```python
from build123d import *

# Parameters (mm, degrees)
EXTRUDE_1_DEPTH     = 4
SKETCH_2_W          = 5.98
SKETCH_2_H          = 10
EXTRUDE_2_DEPTH     = 4
SKETCH_4_R          = 1
SKETCH_4_W          = 55
SKETCH_4_H          = 8
CUT_EXTRUDE_1_DEPTH = 4
SKETCH_5_R          = 1.6
CUT_EXTRUDE_2_DEPTH = 4
SKETCH_6_W          = 31.5
SKETCH_6_H          = 52
EXTRUDE_3_DEPTH     = 4
SKETCH_7_R          = 1.6
CUT_EXTRUDE_3_DEPTH = 4
SKETCH_8_W          = 13.057041555
SKETCH_8_H          = 52
SKETCH_8_W_2        = 44.99
SKETCH_8_H_2        = 3
EXTRUDE_4_DEPTH     = 4
SKETCH_10_R         = 2.05
CUT_EXTRUDE_4_DEPTH = 10
FILLET_1_R          = 1
FILLET_2_R          = 3
SKETCH_11_W         = 28.99
SKETCH_11_H         = 30
CUT_EXTRUDE_5_DEPTH = 10
EXTRUDE_1_2_DEPTH   = 4
FILLET_3_R          = 2
SKETCH_13_R         = 1.6
EXTRUDE_5_DEPTH     = 4
SKETCH_15_R         = 1.6
CUT_EXTRUDE_6_DEPTH = 4


with BuildPart() as part:
    # 草图1 → Extrude 1 (new body)
    with BuildSketch(Plane(origin=(0, 0, 0), x_dir=(1, 0, 0), z_dir=(0, 1, 0))):
        Polygon((-14.01, 30), (-27.5, 30), (-27.5, -30), (27.5, -30), (27.5, 30), (14.01, 30), (14.01, 22), (14.01, -22), (-14.01, -22), (-14.01, 22), align=None)
    extrude(amount=EXTRUDE_1_DEPTH)

    # 草图2 → 凸台-拉伸2 (add)
    with BuildSketch(Plane(origin=(0, 4, 0), x_dir=(1, 0, 0), z_dir=(0, 1, 0))):
        with Locations((-6, -17)):
            Rectangle(SKETCH_2_W, SKETCH_2_H)
        with Locations((6, -17)):
            Rectangle(SKETCH_2_W, SKETCH_2_H)
    extrude(amount=-EXTRUDE_2_DEPTH)

    # 草图4 → 切除-拉伸1 (cut)
    with BuildSketch(Plane.XZ):
        with Locations((8.99, 21)):
            Circle(SKETCH_4_R)
        with Locations((14.01, 21)):
            Circle(SKETCH_4_R)
        with Locations((-2.01, 22)):
            Circle(SKETCH_4_R)
        with Locations((2.01, 22)):
            Circle(SKETCH_4_R)
        with Locations((-14.01, 21)):
            Circle(SKETCH_4_R)
        with Locations((-8.99, 21)):
            Circle(SKETCH_4_R)
        with Locations((0, -26)):
            Rectangle(SKETCH_4_W, SKETCH_4_H)
    extrude(amount=-CUT_EXTRUDE_1_DEPTH, mode=Mode.SUBTRACT)

    # 草图5 → 切除-拉伸2 (cut)
    with BuildSketch(Plane.XZ):
        with Locations(Location((17.01, 10, 0), (0, 0, 270))):
            Circle(SKETCH_5_R)
        with Locations(Location((17.01, -10, 0), (0, 0, 270))):
            Circle(SKETCH_5_R)
        with Locations(Location((-17.01, -10, 0), (0, 0, 270))):
            Circle(SKETCH_5_R)
        with Locations(Location((-17.01, 10, 0), (0, 0, 270))):
            Circle(SKETCH_5_R)
    extrude(amount=-CUT_EXTRUDE_2_DEPTH, mode=Mode.SUBTRACT)

    # 草图6 → 凸台-拉伸3 (add)
    with BuildSketch(Plane.XZ):
        with Locations((43.25, 4)):
            Rectangle(SKETCH_6_W, SKETCH_6_H)
    extrude(amount=-EXTRUDE_3_DEPTH)

    # 草图7 → 切除-拉伸3 (cut)
    with BuildSketch(Plane.XZ):
        with Locations(Location((56, 20, 0), (0, 0, 270))):
            Circle(SKETCH_7_R)
        with Locations(Location((56, 0, 0), (0, 0, 270))):
            Circle(SKETCH_7_R)
    extrude(amount=-CUT_EXTRUDE_3_DEPTH, mode=Mode.SUBTRACT)

    # 草图8 → 凸台-拉伸4 (add)
    with BuildSketch(Plane.XZ):
        with Locations((-34.028520778, 4)):
            Rectangle(SKETCH_8_W, SKETCH_8_H)
        Polygon((-14.01, -25), (-14.01, -22), (-27.5, -22), (-40.557041555, -22), (-40.557041555, -25), align=None)
        with Locations((36.505, -23.5)):
            Rectangle(SKETCH_8_W_2, SKETCH_8_H_2)
    extrude(amount=-EXTRUDE_4_DEPTH)

    # 草图10 → 切除-拉伸4 (cut)
    with BuildSketch(Plane.XZ):
        with Locations(Location((-35.507041555, -20.5, 0), (0, 0, 270))):
            Circle(SKETCH_10_R)
        with Locations(Location((-35.507041555, 20.5, 0), (0, 0, 270))):
            Circle(SKETCH_10_R)
        with Locations(Location((35.507041555, 20.5, 0), (0, 0, 270))):
            Circle(SKETCH_10_R)
        with Locations(Location((35.507041555, -20.5, 0), (0, 0, 270))):
            Circle(SKETCH_10_R)
    extrude(amount=-CUT_EXTRUDE_4_DEPTH, mode=Mode.SUBTRACT)

    # 圆角1
    fillet_1_edges = [part.edges().sort_by_distance(p)[0] for p in [
        (-8.99, 2, 12),
        (-3.01, 2, 12),
        (3.01, 2, 12),
        (8.99, 2, 12),
    ]]
    fillet(fillet_1_edges, radius=FILLET_1_R)

    # 圆角2
    fillet_2_edges = [part.edges().sort_by_distance(p)[0] for p in [
        (59, 2, 30),
        (-40.557041555, 2, -25),
        (-14.01, 2, -25),
        (-40.557041555, 2, 30),
        (14.01, 2, -25),
        (59, 2, -25),
    ]]
    fillet(fillet_2_edges, radius=FILLET_2_R)

    # 草图11 → 切除-拉伸5 (cut)
    with BuildSketch(Plane(origin=(0, 4, 0), x_dir=(1, 0, 0), z_dir=(0, 1, 0))):
        with Locations((36.505, 0)):
            Rectangle(SKETCH_11_W, SKETCH_11_H)
        with BuildLine():
            Line((-23, 11), (-23, -11))
            ThreePointArc((-23, -11), (-28, -16), (-33, -11))
            Line((-33, -11), (-33, 11))
            ThreePointArc((-33, 11), (-28, 16), (-23, 11))
        make_face()
    extrude(amount=-CUT_EXTRUDE_5_DEPTH, mode=Mode.SUBTRACT)

    # 草图12 → Extrude 1 2 (add)
    with BuildSketch(Plane(origin=(0, 4, 0), x_dir=(1, 0, 0), z_dir=(0, 1, 0))):
        Polygon((20.571783704, 13.610203653), (49.561783704, -16.389796347), (52.438216296, -13.610203653), (23.448216296, 16.389796347), align=None)
        Polygon((23.448216296, -16.389796347), (52.438216296, 13.610203653), (49.561783704, 16.389796347), (20.571783704, -13.610203653), align=None)
    extrude(amount=-EXTRUDE_1_2_DEPTH)

    # 圆角3
    fillet_3_edges = [part.edges().sort_by_distance(p)[0] for p in [
        (24.791222833, 2, 15),
        (48.218777167, 2, 15),
        (51, 2, -12.121880477),
        (51, 2, 12.121880477),
        (48.218777167, 2, -15),
        (24.791222833, 2, -15),
        (22.01, 2, 12.121880477),
        (22.01, 2, -12.121880477),
        (33.723777167, 2, 0),
        (36.505, 2, -2.878119523),
        (39.286222833, 2, 0),
        (36.505, 2, 2.878119523),
    ]]
    fillet(fillet_3_edges, radius=FILLET_3_R)

    # 草图13 → 凸台-拉伸5 (add)
    with BuildSketch(Plane.XZ):
        with Locations((17.01, -10)):
            Circle(SKETCH_13_R)
        with Locations((17.01, 10)):
            Circle(SKETCH_13_R)
        with Locations((-17.01, -10)):
            Circle(SKETCH_13_R)
        with Locations((-17.01, 10)):
            Circle(SKETCH_13_R)
    extrude(amount=-EXTRUDE_5_DEPTH)

    # 草图15 → 切除-拉伸6 (cut)
    with BuildSketch(Plane.XZ):
        with Locations(Location((-17.320508076, -10, 0), (0, 0, 270))):
            Circle(SKETCH_15_R)
        with Locations(Location((-17.320508076, 10, 0), (0, 0, 270))):
            Circle(SKETCH_15_R)
        with Locations(Location((17.320508076, 10, 0), (0, 0, 270))):
            Circle(SKETCH_15_R)
        with Locations(Location((17.320508076, -10, 0), (0, 0, 270))):
            Circle(SKETCH_15_R)
    extrude(amount=-CUT_EXTRUDE_6_DEPTH, mode=Mode.SUBTRACT)


solid = part.part
```
Check sheet for the modelled part. Datum: model origin and axes. Units: mm. A direction names the side the tool comes from. Round coordinates to 2 decimals unless told otherwise and drop trailing zeros. Order: outer loops, then holes, each group sorted by start corner. A loop starts at its lowest first (then second) coordinate and runs counter-clockwise, first axis right, second up. Notation, with made-up numbers: M -6,7.5 L 40,7.5 A21 cw 40,35.5 Z; hole C -16,70.5 d7. An arc over 180 degrees is marked long. Answer in a Markdown table with one row per item.
(1) Section check A-A on z = 0. Record the boundary of the cut face in (x, y), plus the area to 3 significant figures.
Findings:
| item | result |
|---|---|
| outline | M -40.56,0 L -33,0 L -33,4 L -40.56,4 Z; M -23,0 L -14.01,0 L -14.01,4 L -23,4 Z; M 14.01,0 L 22.01,0 L 22.01,4 L 14.01,4 Z; M 32.94,0 L 40.07,0 L 40.07,4 L 32.94,4 Z; M 51,0 L 54.4,0 L 54.4,4 L 51,4 Z; M 57.6,0 L 59,0 L 59,4 L 57.6,4 Z |
| area | 146 mm^2 |
(2) Material ranges on line 1 along X through (y, z) = (1.6, 16.5); line 2 along X through (y, z) = (2.4, 13.5); line 3 along X through (y, z) = (1.55, 10), recorded low to high. Write a range as from..to.
Findings:
| item | result |
|---|---|
| line 1 | x = -40.56..-14.01, -8.99..-3.01, 3.01..8.99, 14.01..59 |
| line 2 | x = -40.56..-32.33, -23.67..-14.01, -8.99..-3.01, 3.01..8.99, 14.01..27.57, 45.44..59 |
| line 3 | x = -40.56..-33, -23..-18.92, -15.72..-14.01, 14.01..15.72, 18.92..29.62, 43.39..59 |
(3) Draft check along Z on faces 1 (the cylindrical face through (37.54, 1.97, 20.77)), 2 (the flat face through (14.01, 2, -1)), 3 (the flat face through (12, 2, 22)). Enter one of: +Z half, -Z half, draft (parallel to the pull), parting line (faces both ways), or undercut.
Findings:
| item | result |
|---|---|
| face 1 | undercut |
| face 2 | draft |
| face 3 | -Z half |
(4) Gauge pin test, flat ends, axial feed: pin 1 (4.5 mm diameter, centred on x = 35.51, z = -20.5, fed in from +Y); pin 2 (2.5 mm diameter, centred on x = -35.51, z = -20.5, fed in from -Y); pin 3 (1.6 mm diameter, centred on x = -0.5, y = 1, fed in from -Z). Record the tip position at first contact, or that the pin passes through.
Findings:
| item | result |
|---|---|
| pin 1 | stops at y = 4 |
| pin 2 | passes through |
| pin 3 | stops at z = 22 |
(5) Section check C-C on y = 3.15. Give the number of separate pieces and of enclosed holes in the cut face, plus the area to 3 significant figures.
Findings:
| item | result |
|---|---|
| separate pieces | 1 |
| enclosed holes | 15 |
| area | 3,330 mm^2 |
(6) Set-up check for faces 4 (the flat face through (9, 2, 30)), 5 (the flat face through (8.99, 2, 17)), 6 (the cylindrical face through (36.483, 1.972, -3.756)): record each of +Z, -Z, +X, -X, +Y, -Y from which the full face is reachable in a straight line by a thin tool's end or side.
Findings:
| item | result |
|---|---|
| face 4 | +Z, +X, -X, +Y, -Y |
| face 5 | -Z, +Y, -Y |
| face 6 | +Y, -Y |
(7) Section check B-B on x = 11.5. Record the boundary of the cut face in (y, z).
Findings:
| item | result |
|---|---|
| outline | M 0,22 L 4,22 L 4,30 L 0,30 Z |
